Source: three-view drawing plus pictorial views. Frame: mm from the lowest corner of the part. Give positions to 0.01 mm unless a question says otherwise; leave off trailing zeros. Loops run counter-clockwise (first coordinate to the right, second up) from the corner with the lowest first, then second, coordinate; pieces in that order, holes last. Notation, with made-up numbers: (24, 29) - (46, 29) arc R16 cw to (46, 42) - close; hole circle Ø3 at (49.5, 54.25). An arc over 180 degrees is marked (long way). Write each question's results on one line, items separated by ' | '. Start each with the question number.
(1) Material intervals for line 1 along X through (y, z) = (8, 211.5); line 2 along Y through (x, z) = (27, 210.5); line 3 along Y through (x, z) = (171.5, 33), sorted ascending. Write a range as [from, to].
(2) Pull-direction query (X, two-part tool) for the marked faces 1 and 2; classes: pulls with the +X half, pulls with the -X half, needs draft (parallel to the pull), parting line crosses it, or undercut.
(3) Cut plane A-A on y = 12. Return the cut outline in (x, z), then the cut area to 3 significant figures.
(4) Cut plane B-B on z = 70. Return the cut outline in (x, y).
(5) Cut plane C-C on x = 126.5. Return the cut outline in (y, z).
(6) Contact query for flat-ended pins moving along their axis: pin 1 (8 mm diameter, centred on y = 11.5, z = 51.5, fed in from -X); pin 2 (2 mm diameter, centred on x = 150.5, z = 268.5, fed in from -Y); pin 3 (18.5 mm diameter, centred on x = 11.5, z = 113, fed in from +Y); pin 4 (8 mm diameter, centred on x = 150, y = 11, fed in from -Z). Output: stop coordinate, or through.
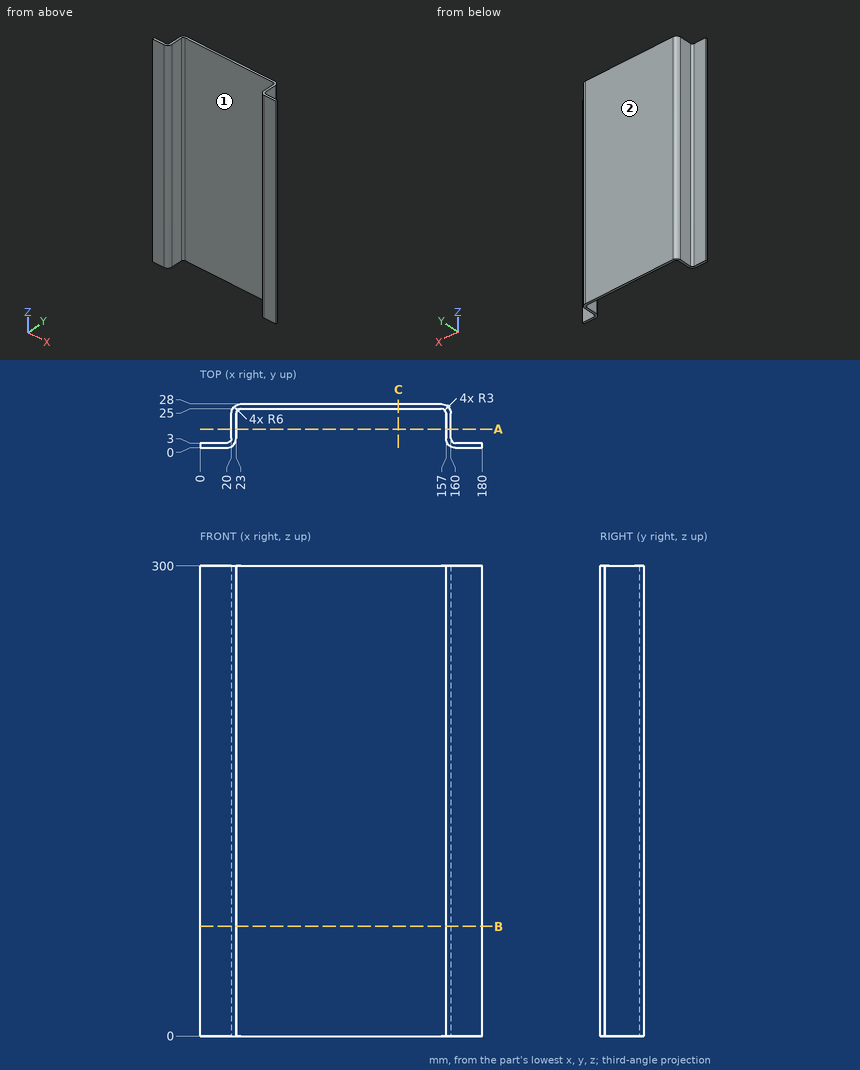
Ans:
1) line 1: [20, 23], [157, 160] | line 2: [25, 28] | line 3: [0, 3]
2) face 1: undercut | face 2: needs draft
3) outline: (20, 0) - (23, 0) - (23, 300) - (20, 300) - close; (157, 0) - (160, 0) - (160, 300) - (157, 300) - close | area: 1,800 mm^2
4) outline: (0, 0) - (17, 0) arc R6 ccw to (23, 6) - (23, 22) arc R3 cw to (26, 25) - (154, 25) arc R3 cw to (157, 22) - (157, 6) arc R6 ccw to (163, 0) - (180, 0) - (180, 3) - (163, 3) arc R3 cw to (160, 6) - (160, 22) arc R6 ccw to (154, 28) - (26, 28) arc R6 ccw to (20, 22) - (20, 6) arc R3 cw to (17, 3) - (0, 3) - close
5) outline: (25, 0) - (28, 0) - (28, 300) - (25, 300) - close
6) pin 1: x = 20 | pin 2: y = 25 | pin 3: y = 24.9 | pin 4: through
